Part model, mm, in its own coordinate system. A direction names the side the tool comes from. Give positions to 0.01 mm unless a question says otherwise; leave off trailing zeros. Order: outer loops, then holes, each group sorted by start corner. A loop starts at its lowest first (then second) coordinate and runs counter-clockwise, first axis right, second up. Notation, with made-up numbers: (-1.75, -29) - (51.25, -29) arc R34 ccw to (51.25, 3) - close; hole circle Ø10 at (2.5, -4.75). An arc over 180 degrees is marked (long way). One line per item, written item: value.
```python
from build123d import *

# Parameters (mm, degrees)
SKETCH1_W           = 42
SKETCH1_H           = 64
BOSS_EXTRUDE1_DEPTH = 20
SKETCH4_W           = 42
SKETCH4_H           = 29
BOSS_EXTRUDE2_DEPTH = 3
SKETCH5_W           = 9
SKETCH5_H           = 19
CUT_EXTRUDE1_DEPTH  = 4
CUT_EXTRUDE2_REACH  = 50.154
CUT_EXTRUDE2_START  = 3.5
SKETCH6_W           = 5
SKETCH6_H           = 5
FILLET1_R           = 3
FILLET2_R           = 1
SKETCH7_R           = 1.471142405
SKETCH7_R_2         = 1.415504474
CUT_EXTRUDE3_DEPTH  = 43.956373217
SKETCH8_W           = 21
SKETCH8_H           = 21.4
SKETCH8_W_2         = 20
SKETCH8_H_2         = 21
SKETCH8_R           = 1
CUT_EXTRUDE5_DEPTH  = 4
SKETCH10_W          = 11
SKETCH10_H          = 4.5
CUT_EXTRUDE6_DEPTH  = 4


with BuildPart() as part:
    # Sketch1 → Boss-Extrude1 (new body)
    with BuildSketch(Plane(origin=(0, 0, 0), x_dir=(1, 0, 0), z_dir=(0, 1, 0))):
        Rectangle(SKETCH1_W, SKETCH1_H)
    extrude(amount=BOSS_EXTRUDE1_DEPTH)

    # Sketch4 → Boss-Extrude2 (add)
    with BuildSketch(Plane(origin=(0, 20, 0), x_dir=(1, 0, 0), z_dir=(0, 1, 0))):
        with Locations((0, 17.5)):
            Rectangle(SKETCH4_W, SKETCH4_H)
    extrude(amount=BOSS_EXTRUDE2_DEPTH)

    # Sketch5 → Cut-Extrude1 (cut)
    with BuildSketch(Plane(origin=(0, 20, 0), x_dir=(1, 0, 0), z_dir=(0, 1, 0))):
        with Locations((16.5, -6.5)):
            Rectangle(SKETCH5_W, SKETCH5_H)
    extrude(amount=-CUT_EXTRUDE1_DEPTH, mode=Mode.SUBTRACT)

    # Sketch6 → Cut-Extrude2 (cut, up to next)
    with BuildSketch(Plane(origin=(0, 0, 0), x_dir=(1, 0, 0), z_dir=(0, 1, 0)).offset(CUT_EXTRUDE2_START), mode=Mode.PRIVATE) as cut_extrude2_sk1:
        with Locations((-18.5, 29.5)):
            Rectangle(SKETCH6_W, SKETCH6_H)
    cut_extrude2_tool1 = extrude(cut_extrude2_sk1.sketch, amount=CUT_EXTRUDE2_REACH, mode=Mode.PRIVATE) & part.part
    # Sketch6 → Cut-Extrude2 (cut, up to next)
    with BuildSketch(Plane(origin=(0, 0, 0), x_dir=(1, 0, 0), z_dir=(0, 1, 0)).offset(CUT_EXTRUDE2_START), mode=Mode.PRIVATE) as cut_extrude2_sk2:
        with Locations((18.5, -29.5)):
            Rectangle(SKETCH6_W, SKETCH6_H)
    cut_extrude2_tool2 = extrude(cut_extrude2_sk2.sketch, amount=CUT_EXTRUDE2_REACH, mode=Mode.PRIVATE) & part.part
    add(cut_extrude2_tool1.solids().sort_by_distance((-18.5, 3.5, -29.5))[0], mode=Mode.SUBTRACT)
    add(cut_extrude2_tool2.solids().sort_by_distance((18.5, 3.5, 29.5))[0], mode=Mode.SUBTRACT)

    # Fillet1
    fillet1_edges = [part.edges().sort_by_distance(p)[0] for p in [
        (-16, 13.25, -27),
        (16, 11.75, 27),
    ]]
    fillet(fillet1_edges, radius=FILLET1_R)

    # Fillet2
    fillet2_edges = [part.edges().sort_by_distance(p)[0] for p in [
        (21, 1.75, 32),
        (-21, 1.75, -32),
        (-21, 13.25, -27),
        (-16, 13.25, -32),
        (21, 11.5, -32),
        (-21, 10, 32),
        (16, 11.75, 32),
        (21, 11.75, 27),
        (0, 23, -3),
        (-21, 23, -15),
    ]]
    fillet(fillet2_edges, radius=FILLET2_R)

    # Sketch7 → Cut-Extrude3 (cut, through all)
    with BuildSketch(Plane(origin=(0, 3.5, 0), x_dir=(1, 0, 0), z_dir=(0, 1, 0))):
        with Locations(Location((18.5, -29.5, 0), (0, 0, 270))):
            Circle(SKETCH7_R)
        with Locations(Location((-18.5, 29.5, 0), (0, 0, 270))):
            Circle(SKETCH7_R_2)
    extrude(amount=-CUT_EXTRUDE3_DEPTH, mode=Mode.SUBTRACT)

    # Sketch8 → Cut-Extrude5 (cut)
    # profile 1 of 7: a face of its own
    with BuildSketch(Plane(origin=(21, 0, 0), x_dir=(0, 0, -1), z_dir=(1, 0, 0))):
        with Locations((15, 11.5)):
            Rectangle(SKETCH8_W, SKETCH8_H)
        with Locations((15, 11.5)):
            Rectangle(SKETCH8_W_2, SKETCH8_H_2, mode=Mode.SUBTRACT)
    # profile 2 of 7: a face of its own
    with BuildSketch(Plane(origin=(21, 0, 0), x_dir=(0, 0, -1), z_dir=(1, 0, 0))):
        with Locations((23, 20)):
            Circle(SKETCH8_R)
    # profile 3 of 7: a face of its own
    with BuildSketch(Plane(origin=(21, 0, 0), x_dir=(0, 0, -1), z_dir=(1, 0, 0))):
        with BuildLine():
            ThreePointArc((19.415599916, 19.911449184), (17.273898937, 20.723848634), (15, 21))
            Line((15, 21), (15, 17.5))
            ThreePointArc((15, 17.5), (16.160499883, 17.386700266), (17.277171656, 17.051080008))
            Line((17.277171656, 17.051080008), (19.415599916, 19.911449184))
        make_face()
    # profile 4 of 7: a face of its own
    with BuildSketch(Plane(origin=(21, 0, 0), x_dir=(0, 0, -1), z_dir=(1, 0, 0))):
        with BuildLine():
            Line((15, 17.5), (15, 21))
            ThreePointArc((15, 21), (7.742797617, 17.63049864), (5.633627508, 9.912213384))
            Line((5.633627508, 9.912213384), (9.02780956, 10.922989297))
            ThreePointArc((9.02780956, 10.922989297), (10.558037359, 15.533480865), (15, 17.5))
        make_face()
    # profile 5 of 7: a face of its own
    with BuildSketch(Plane(origin=(21, 0, 0), x_dir=(0, 0, -1), z_dir=(1, 0, 0))):
        with BuildLine():
            ThreePointArc((6.000737249, 8.456437952), (9.462123126, 3.781067449), (15, 2))
            Line((15, 2), (15, 5.5))
            ThreePointArc((15, 5.5), (11.554812633, 6.587700741), (9.358736217, 9.456438665))
            Line((9.358736217, 9.456438665), (6.000737249, 8.456437952))
        make_face()
    # profile 6 of 7: a face of its own
    with BuildSketch(Plane(origin=(21, 0, 0), x_dir=(0, 0, -1), z_dir=(1, 0, 0))):
        with BuildLine():
            Line((15, 5.5), (15, 2))
            ThreePointArc((15, 2), (18.598182651, 2.707782896), (21.660211168, 4.725667029))
            Line((21.660211168, 4.725667029), (19.206449159, 7.221473913))
            ThreePointArc((19.206449159, 7.221473913), (17.272536411, 5.947020776), (15, 5.5))
        make_face()
    # profile 7 of 7: a face of its own
    with BuildSketch(Plane(origin=(21, 0, 0), x_dir=(0, 0, -1), z_dir=(1, 0, 0))):
        with BuildLine():
            Line((20.142508406, 8.40894722), (22.646296664, 5.862256894))
            ThreePointArc((22.646296664, 5.862256894), (24.397892993, 12.889103053), (20.688333963, 19.108735554))
            Line((20.688333963, 19.108735554), (18.592631977, 16.305517192))
            ThreePointArc((18.592631977, 16.305517192), (20.887667085, 12.655584827), (20.142508406, 8.40894722))
        make_face()
    extrude(amount=-CUT_EXTRUDE5_DEPTH, mode=Mode.SUBTRACT)

    # Sketch10 → Cut-Extrude6 (cut)
    with BuildSketch(Plane.ZY.offset(21)):
        with Locations((-16.5, 17.75)):
            Rectangle(SKETCH10_W, SKETCH10_H)
    extrude(amount=-CUT_EXTRUDE6_DEPTH, mode=Mode.SUBTRACT)


solid = part.part
```
1) Slice it at B-B on z = 1. Write the cut outline in (x, y).
Answer:
outline: (-21, 0) - (21, 0) - (21, 16) - (12, 16) - (12, 20) - (-21, 20) - close
2) Wall check: line 1 along X through (y, z) = (2.55, 29.5); line 2 along Y through (x, z) = (-11.5, 27); line 3 along X through (y, z) = (2.3, -29.5). Give the ranges that are in metal, low to high. Write a range as [from, to].
Answer:
line 1: x = [-21, 17.03], [19.97, 21]
line 2: y = [0, 20]
line 3: x = [-21, -19.92], [-17.08, 21]
3) Slice it at A-A on x = -14. Write the cut outline in (y, z), then the cut area to 3 significant figures.
Answer:
outline: (0, -32) - (23, -32) - (23, -4) arc R1 ccw to (22, -3) - (20, -3) - (20, 32) - (0, 32) - close
area: 1,370 mm2
4) Two-plate mould, pull along X, no slides. Class faces 5 (the face through (-16.9, 13.39, -27.86)), 6 (the face through (19, 19, -23)), 7 (the face through (17.064, 1.774, 29.181)): pulls with the +X half, pulls with the -X half, needs draft (parallel to the pull), parting line crosses it, or undercut.
Answer:
face 5: pulls with the -X half
face 6: needs draft
face 7: undercut
5) Which spindle directions (+Z, -Z, +X, -X, +Y, -Y) get a long thin tool onto all of the face, cutting with end or side? Do faces 1 (the face through (-19, 15.5, -17)), 2 (the face through (16, 16, 6)), 3 (the face through (19.028, 5.956, -20.451)), 4 (the face through (0, 10, 32)). Say none if no direction does.
Answer:
face 1: -X
face 2: +X, +Y
face 3: +X
face 4: +Z, +X, -X, +Y, -Y
6) Drop flat-ended pins along their axis: P1, Ø4.5, axis at x = 19, y = 9.5, coming from the +Z side; P2, Ø0.8, axis at x = 19.5, y = 15, coming from the +Z side; P3, Ø1.2, axis at y = 18.5, z = 10, coming from the +X side. Give the stop position or say it passes through.
Answer:
P1: stops at z = 28.02
P2: stops at z = 27
P3: stops at x = 12
